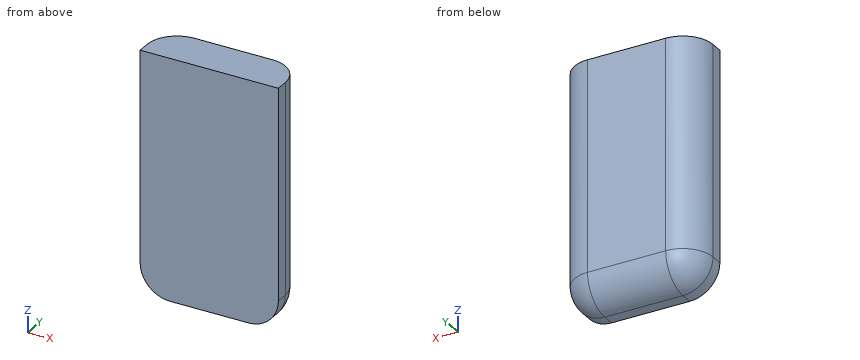
```python
from build123d import *

# Parameters (mm, degrees)
SKETCH1_W           = 23
SKETCH1_H           = 40
BOSS_EXTRUDE1_DEPTH = 7
FILLET1_R           = 5
FILLET2_R           = 5
FILLET3_R           = 5


with BuildPart() as part:
    # Sketch1 → Boss-Extrude1 (new body)
    with BuildSketch(Plane(origin=(0, 0, 0), x_dir=(1, 0, 0), z_dir=(0, 1, 0))):
        Rectangle(SKETCH1_W, SKETCH1_H)
    extrude(amount=BOSS_EXTRUDE1_DEPTH)

    # Fillet1
    fillet1_edges = [part.edges().sort_by_distance(p)[0] for p in [
        (-11.5, 3.5, -20),
    ]]
    fillet(fillet1_edges, radius=FILLET1_R)

    # Fillet2
    fillet2_edges = [part.edges().sort_by_distance(p)[0] for p in [
        (11.5, 3.5, -20),
    ]]
    fillet(fillet2_edges, radius=FILLET2_R)

    # Fillet3
    fillet3_edges = [part.edges().sort_by_distance(p)[0] for p in [
        (-11.5, 7, 2.5),
        (-10.035533906, 7, -18.535533906),
        (0, 7, -20),
        (10.035533906, 7, -18.535533906),
        (11.5, 7, 2.5),
    ]]
    fillet(fillet3_edges, radius=FILLET3_R)


solid = part.part
```
CAD build for the part. Positions are in the model's coordinates, mm. Round coordinates to 2 decimals unless told otherwise and drop trailing zeros. Order: outer loops, then holes, each group sorted by start corner. A loop starts at its lowest first (then second) coordinate and runs counter-clockwise, first axis right, second up. Notation, with made-up numbers: (-13, 89) - (29, 89) arc R13 cw to (29, 114) - close; hole circle Ø5 at (31, -3). An arc over 180 degrees is marked (long way). Answer as CSV lines item,"result". Start each with the question number.
1. Drill centre lines: L1, parallel to Z at x = -7, y = 4.5; L2, parallel to X at y = 3.75, z = 7; L3, parallel to Y at x = 0.75, z = -17. Where is each one in solid material? Low to high. Write a range as [from, to].
2. Saw through at B-B, the plane z = -11. Write the cut outline in (x, y), and give its area (3 significant figures).
3. Saw through at A-A, the plane y = 6. Write the cut outline in (x, z).
4. Saw through at C-C, the plane x = -3.75. Write the cut outline in (y, z), and give its area (3 significant figures).
5. Pin check, flat tip, straight feed: pin 1 (1.5 mm diameter, centred on y = 5, z = -2.5, fed in from -X). Stop position of the tip, or through.
6. Saw through at D-D, the plane x = 9. Write the cut outline in (y, z), and give its area (3 significant figures).
Model answer:
1,L1,"z = [-19.3, 20]"
1,L2,"x = [-11.18, 11.18]"
1,L3,"y = [0, 6.58]"
2,outline,"(-11.5, 0) - (11.5, 0) - (11.5, 2) arc R5 ccw to (6.5, 7) - (-6.5, 7) arc R5 ccw to (-11.5, 2) - close"
2,area,"150 mm²"
3,outline,"(-9.5, -15) arc R3 ccw to (-6.5, -18) - (6.5, -18) arc R3 ccw to (9.5, -15) - (9.5, 20) - (-9.5, 20) - close"
4,outline,"(0, -20) - (2, -20) arc R5 ccw to (7, -15) - (7, 20) - (0, 20) - close"
4,area,"275 mm²"
5,pin 1,"stops at x = -10.97"
6,outline,"(0, -19.33) - (2, -19.33) arc R4.33 ccw to (6.33, -15) - (6.33, 20) - (0, 20) - close"
6,area,"245 mm²"
